```python
from build123d import *

# Parameters (mm, degrees)
BOSS_EXTRUDE1_DEPTH                                  = 2
EXTRUDE_THIN2_DEPTH                                  = 19.5
CHAMFER1_SIZE                                        = 1.5
CSK_FOR_ST2_2_CROSS_RECESSED_CTSK_HEAD_T_D           = 2.8
CSK_FOR_ST2_2_CROSS_RECESSED_CTSK_HEAD_T_DEPTH       = 7.5
CSK_FOR_ST2_2_CROSS_RECESSED_CTSK_HEAD_T_CSINK_D     = 4.8
CSK_FOR_ST2_2_CROSS_RECESSED_CTSK_HEAD_T_CSINK_ANGLE = 90
CSK_FOR_ST2_2_CROSS_RECESSED_CTSK_HEAD_T_TIP         = 0.841204867
SKETCH4_R                                            = 5.75
SKETCH4_R_2                                          = 4.25
EXTRUDE_THIN1_DEPTH                                  = 0.5


with BuildPart() as part:
    # Sketch1 → Boss-Extrude1 (new body)
    with BuildSketch(Plane.XZ.offset(-2)):
        with BuildLine():
            Line((0, -27.9), (20, -27.9))
            ThreePointArc((20, -27.9), (47.9, 0), (20, 27.9))
            Line((20, 27.9), (0, 27.9))
            ThreePointArc((0, 27.9), (-27.9, 0), (0, -27.9))
        make_face()
    extrude(amount=BOSS_EXTRUDE1_DEPTH)

    # Sketch8 → Extrude-Thin2 (add)
    with BuildSketch(Plane(origin=(0, 2, 0), x_dir=(1, 0, 0), z_dir=(0, 1, 0))):
        with BuildLine():
            ThreePointArc((33.69302994, -9.206026887), (24.155985639, -15.968023778), (12.53247907, -14.71346768))
            Line((12.53247907, -14.71346768), (11.401036505, -16.942780965))
            ThreePointArc((11.401036505, -16.942780965), (24.785680433, -18.38742132), (35.767731446, -10.600879446))
            Line((35.767731446, -10.600879446), (33.69302994, -9.206026887))
        make_face()
    extrude(amount=EXTRUDE_THIN2_DEPTH)

    # Chamfer1
    chamfer1_edges = [part.edges().sort_by_distance(p)[0] for p in [
        (24.155985639, 2, 15.968023778),
        (24.785680433, 2, 18.38742132),
    ]]
    chamfer(chamfer1_edges, length=CHAMFER1_SIZE)

    # CSK for ST2.2 Cross recessed CTSK head tapping screws1
    with Locations(Plane(origin=(0, 0, 0), x_dir=(-1, 0, 0), z_dir=(0, -1, 0))):
        with Locations((-39, 16), (-39, -16), (19, -16), (19, 16)):
            CounterSinkHole(CSK_FOR_ST2_2_CROSS_RECESSED_CTSK_HEAD_T_D / 2, CSK_FOR_ST2_2_CROSS_RECESSED_CTSK_HEAD_T_CSINK_D / 2, depth=CSK_FOR_ST2_2_CROSS_RECESSED_CTSK_HEAD_T_DEPTH, counter_sink_angle=CSK_FOR_ST2_2_CROSS_RECESSED_CTSK_HEAD_T_CSINK_ANGLE)
            with Locations((0, 0, -(CSK_FOR_ST2_2_CROSS_RECESSED_CTSK_HEAD_T_DEPTH + CSK_FOR_ST2_2_CROSS_RECESSED_CTSK_HEAD_T_TIP / 2))):  # 118° drill point
                Cone(0, CSK_FOR_ST2_2_CROSS_RECESSED_CTSK_HEAD_T_D / 2, CSK_FOR_ST2_2_CROSS_RECESSED_CTSK_HEAD_T_TIP, mode=Mode.SUBTRACT)

    # Sketch4 → Extrude-Thin1 (add)
    with BuildSketch(Plane.XZ):
        with Locations((-11, 19.052558883)):
            Circle(SKETCH4_R)
        with Locations((-11, 19.052558883)):
            Circle(SKETCH4_R_2, mode=Mode.SUBTRACT)
        with Locations((-11, -19.052558883)):
            Circle(SKETCH4_R)
        with Locations((-11, -19.052558883)):
            Circle(SKETCH4_R_2, mode=Mode.SUBTRACT)
        with Locations((40.673237657, 7.524443153)):
            Circle(SKETCH4_R)
        with Locations((40.673237657, 7.524443153)):
            Circle(SKETCH4_R_2, mode=Mode.SUBTRACT)
        with Locations((40.673237657, -7.524443153)):
            Circle(SKETCH4_R)
        with Locations((40.673237657, -7.524443153)):
            Circle(SKETCH4_R_2, mode=Mode.SUBTRACT)
    extrude(amount=EXTRUDE_THIN1_DEPTH)


solid = part.part
```
Geometry check sheet. Reference: the model listing, model coordinates, mm. A direction names the side the tool comes from. Round coordinates to 2 decimals unless told otherwise and drop trailing zeros. Order: outer loops, then holes, each group sorted by start corner. A loop starts at its lowest first (then second) coordinate and runs counter-clockwise, first axis right, second up. Notation, with made-up numbers: (42.25, 42) -> (61.25, 42) arc R26 cw to (61.25, 76) -> close; hole circle Ø6 at (71.5, 23.25). An arc over 180 degrees is marked (long way). Return JSON: item names as keys, results as strings. Group by question number.
Q1. Tool access check on faces 1 (the conical face through (24.66, 3.26, 18.67)), 2 (the flat face through (11.984, 11.613, 15.794)), 3 (the cylindrical face through (46.16, -0.25, -5.8)). Record the directions out of +Z, -Z, +X, -X, +Y, -Y that give a thin tool (end or side, any length) a straight path to the whole face; none if there is none.
Q2. Section check C-C, the plane z = 0. Record the boundary of the cut face in (x, y), plus the area to 3 significant figures.
Q3. Section check A-A, the plane x = -11. Record the boundary of the cut face in (y, z).
Q4. Section check B-B, the plane x = 39. Count the separate pieces of the cut face and the enclosed holes in it, plus the area to 3 significant figures.
Q5. Section check D-D, the plane y = 13. Record the boundary of the cut face in (x, z), plus the area to 3 significant figures.
Q6. Gauge pin test, flat ends, axial feed: pin 1 (2.5 mm diameter, centred on x = 42.5, z = 7.5, fed in from -Y); pin 2 (8 mm diameter, centred on y = 7.5, z = 1, fed in from +X); pin 3 (16.5 mm diameter, centred on x = 24.5, z = -10.5, fed in from +Y); pin 4 (11 mm diameter, centred on x = -11, z = 19.05, fed in from -Y). Record the tip position at first contact, or that the pin passes through.
Q7. Material ranges on probe 1 along Z at (x, y) = (39, 1.35); probe 2 along Y at (x, z) = (-1, -2); probe 3 along Z at (x, y) = (20.5, 1.25), recorded low to high. Write a range as from..to.
Q8. Release check for a two-part mould opening along Z. For faces 4 (the cylindrical face through (24.599, 12.374, 18.435)), 5 (the cylindrical face through (39.75, 1.51, 14.82)), 6 (the flat face through (24.4, 21.5, 16.3)) record: released by +Z, released by -Z, zero draft, split by the parting line, or undercut.
Numbers:
{
 "1": {"face 1": "+Z, +Y", "face 2": "-Z, -X, +Y", "face 3": "-Y"},
 "2": {"outline": "(-27.9, 0) -> (47.9, 0) -> (47.9, 2) -> (-27.9, 2) -> close", "area": "152 mm^2"},
 "3": {"outline": "(-0.5, -24.8) -> (0, -24.8) -> (0, -25.64) -> (2, -25.64) -> (2, 25.64) -> (0, 25.64) -> (0, 24.8) -> (-0.5, 24.8) -> (-0.5, 23.3) -> (0, 23.3) -> (0, 14.8) -> (-0.5, 14.8) -> (-0.5, 13.3) -> (0, 13.3) -> (0, -13.3) -> (-0.5, -13.3) -> (-0.5, -14.8) -> (0, -14.8) -> (0, -23.3) -> (-0.5, -23.3) -> close"},
 "4": {"separate pieces": "3", "enclosed holes": "0", "area": "71.7 mm^2"},
 "5": {"outline": "(11.4, 16.94) -> (12.53, 14.71) arc R16.5 cw to (33.69, 9.21) -> (35.77, 10.6) arc R19 ccw to start", "area": "64.3 mm^2"},
 "6": {"pin 1": "y = 0", "pin 2": "through", "pin 3": "y = 2", "pin 4": "y = -0.5"},
 "7": {"probe 1": "-20.43..-17.4, -14.6..14.6, 17.4..20.43", "probe 2": "0..2", "probe 3": "-27.9..27.9"},
 "8": {"face 4": "released by +Z", "face 5": "undercut", "face 6": "zero draft"}
}
